Here's how the part is built. I have some questions about the finished solid (model axes, mm). Face numbers are marked on the shaded views. A direction names the side the tool comes from. Coordinates: 2 decimals unless noted, no trailing zeros. Write each loop counter-clockwise with the first axis right and the second up, starting at its lowest first coordinate (ties: lowest second). Pieces come first, ordered by that corner, then holes.
(1) Imagine slicing it at A-A, the plane x = 42. List the corners of the cut face in (y, z) for me, plus the area to 3 significant figures.
(2) Imagine slicing it at C-C, the plane z = -7.75. State how many separate pieces and enclosed holes the cut face has, plus the area to 3 significant figures.
(3) Which directions (+Z, -Z, +X, -X, +Y, -Y) give clear straight access to the entire face, cutting with the end or side of a thin tool? Please do the marked faces 4, 5 and 6.
(4) Please list where these lines run through material, in increasing order: probe 1 along X at (y, z) = (6.25, -4); probe 2 along X at (y, z) = (12, -4.75); probe 3 along Y at (x, z) = (3, -4.5).
(5) For pin 1 Ø2 at (y, z) = (19, -7.5) entering from +X; pin 2 Ø7.5 at (y, z) = (16, -10.5) entering from -X; pin 3 Ø3 at (x, z) = (4, -5) entering from +Y; pin 4 Ø5 at (x, y) = (15, 20) entering from +Z, each with a flat end and sliding along its axis, tell me the tip position at first contact or that it passes through.
(6) Thinking about a two-plate mould opening in X: for the marked faces 1, 2 and 3, which applies, released by +X, released by -X, zero draft, split by the parting line, or undercut?
(7) Imagine slicing it at B-B, the plane z = -3. List the corners of the cut face in (x, y) for me, plus the area to 3 significant figures.
(8) Imagine slicing it at D-D, the plane x = 7. List the corners of the cut face in (y, z) for me, plus the area to 3 significant figures.
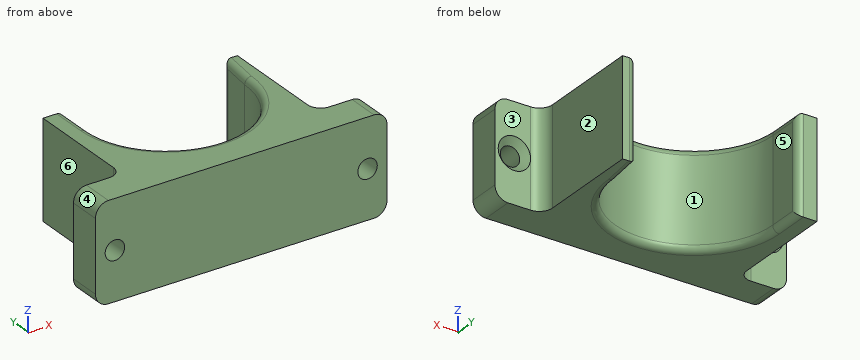
```python
from build123d import *

# Parameters (mm, degrees)
SKETCH1_W           = 45
SKETCH1_H           = 15
BOSS_EXTRUDE1_DEPTH = 5
SKETCH2_W           = 30
SKETCH2_H           = 15
BOSS_EXTRUDE2_DEPTH = 18
FILLET1_R           = 2
SKETCH3_R           = 1.5
CUT_EXTRUDE1_DEPTH  = 20
CHAMFER1_SIZE       = 1
CUT_EXTRUDE2_DEPTH  = 20
CUT_EXTRUDE3_DEPTH  = 20
FILLET2_R           = 1


with BuildPart() as part:
    # Sketch1 → Boss-Extrude1 (new body)
    with BuildSketch(Plane(origin=(0, 0, 0), x_dir=(1, 0, 0), z_dir=(0, 1, 0))):
        with Locations((22.5, 7.5)):
            Rectangle(SKETCH1_W, SKETCH1_H)
    extrude(amount=BOSS_EXTRUDE1_DEPTH)

    # Sketch2 → Boss-Extrude2 (add)
    with BuildSketch(Plane(origin=(0, 5, 0), x_dir=(1, 0, 0), z_dir=(0, 1, 0))):
        with Locations((22.5, 7.5)):
            Rectangle(SKETCH2_W, SKETCH2_H)
    extrude(amount=BOSS_EXTRUDE2_DEPTH)

    # Fillet1
    fillet1_edges = [part.edges().sort_by_distance(p)[0] for p in [
        (7.5, 5, -7.5),
        (37.5, 5, -7.5),
        (0, 2.5, 0),
        (0, 2.5, -15),
        (45, 2.5, -15),
        (45, 2.5, 0),
    ]]
    fillet(fillet1_edges, radius=FILLET1_R)

    # Sketch3 → Cut-Extrude1 (cut)
    with BuildSketch(Plane(origin=(0, 5, 0), x_dir=(1, 0, 0), z_dir=(0, 1, 0))):
        with Locations(Location((3, 7.524826623, 0), (0, 0, 270))):
            Circle(SKETCH3_R)
        with Locations(Location((42, 7.524826623, 0), (0, 0, 270))):
            Circle(SKETCH3_R)
    extrude(amount=-CUT_EXTRUDE1_DEPTH, mode=Mode.SUBTRACT)

    # Chamfer1
    chamfer1_edges = [part.edges().sort_by_distance(p)[0] for p in [
        (3, 5, -9.024826623),
        (42, 5, -9.024826623),
    ]]
    chamfer(chamfer1_edges, length=CHAMFER1_SIZE - 0.0001)  # a hair under: the kernel refuses the full size

    # Sketch4 → Cut-Extrude2 (cut)
    with BuildSketch(Plane.XY):
        with BuildLine():
            Line((11.916858064, 23), (33.584575987, 23))
            ThreePointArc((33.584575987, 23), (22.750717026, 5.35), (11.916858064, 23))
        make_face()
    extrude(amount=-CUT_EXTRUDE2_DEPTH, mode=Mode.SUBTRACT)

    # Sketch6 → Cut-Extrude3 (cut)
    with BuildSketch(Plane.XY):
        with BuildLine():
            ThreePointArc((33.584575987, 23), (34.567101549, 20.327641563), (34.900717026, 17.5))
            Line((34.900717026, 17.5), (35.542287994, 23))
            Line((35.542287994, 23), (33.584575987, 23))
        make_face()
        with BuildLine():
            Line((10.600717026, 23), (10.600717026, 17.5))
            ThreePointArc((10.600717026, 17.5), (10.934332503, 20.327641563), (11.916858064, 23))
            Line((11.916858064, 23), (10.600717026, 23))
        make_face()
    extrude(amount=-CUT_EXTRUDE3_DEPTH, mode=Mode.SUBTRACT)

    # Fillet2
    fillet2_edges = [part.edges().sort_by_distance(p)[0] for p in [
        (22.750717026, 5.35, 0),
        (22.750717026, 5.35, -15),
        (35.22150251, 20.25, -15),
        (35.542287994, 23, -7.5),
        (35.22150251, 20.25, 0),
        (10.600717026, 23, -7.5),
        (10.600717026, 20.25, -15),
        (10.600717026, 20.25, 0),
    ]]
    fillet(fillet2_edges, radius=FILLET2_R)


solid = part.part
```
Recorded:
1. outline: (0, -15) - (5, -15) - (5, -10.02) - (4, -9.02) - (0, -9.02) - close; (0, -6.02) - (4, -6.02) - (5, -5.02) - (5, 0) - (0, 0) - close
1. area: 59.0 mm2
2. separate pieces: 3
2. enclosed holes: 0
2. area: 367 mm2
3. face 4: +Z, -X, +Y, -Y
3. face 5: +Z, -Z, +Y
3. face 6: +Z, -Z, -X, +Y
4. probe 1: x = 7.35 to 18.16, 27.34 to 37.65
4. probe 2: x = 7.5 to 11.92, 33.58 to 37.5
4. probe 3: y = 0 to 5
5. pin 1: stops at x = 37.5
5. pin 2: stops at x = 7.5
5. pin 3: stops at y = 5
5. pin 4: passes through
6. face 1: undercut
6. face 2: released by +X
6. face 3: zero draft
7. outline: (0, 0) - (45, 0) - (45, 5) - (39.5, 5) arc R2 cw to (37.5, 7) - (37.5, 23) - (36.43, 23) arc R1 ccw to (35.44, 22.12) - (34.9, 17.5) arc R12.15 cw to (10.6, 17.5) - (10.6, 22) arc R1 ccw to (9.6, 23) - (7.5, 23) - (7.5, 7) arc R2 cw to (5.5, 5) - (0, 5) - close
7. area: 399 mm2
8. outline: (0, -15) - (5.68, -15) - (5.68, 0) - (0, 0) - close
8. area: 85.2 mm2
